For this review, take the finished solid that the model builds, in its own axes (mm). A direction names the side the tool comes from. Round coordinates to 2 decimals unless told otherwise and drop trailing zeros. Loops run counter-clockwise (first coordinate to the right, second up) from the corner with the lowest first, then second, coordinate; pieces in that order, holes last.
1) Mouldability with a two-part tool opening along Y and no side actions: class faces 1 (the flat face through (-5, 11, 0)), 2 (the flat face through (5, 20, 4)) as pulls with the +Y half, pulls with the -Y half, needs draft (parallel to the pull), parting line crosses it, or undercut.
2) Take a section at C-C (y = 19). State the section outline as (x, z) points.
3) Take a section at A-A (y = -20). State the section outline as (x, z) points, then the cut area to 3 significant figures.
4) Tool access review of faces 3 (the flat face through (-5, 11, 8)), 4 (the flat face through (-5, 20, 4)): name each direction out of +Z, -Z, +X, -X, +Y, -Y from which nothing blocks a thin tool from reaching the whole face with its end or side.
5) Wall thickness on L1, parallel to X at y = -20, z = 3.5; L2, parallel to Y at x = 0, z = 4.75 (3 decimals); L3, parallel to X at y = -6.5, z = 4.75: over which ranges is each line inside the solid? List them lowest first.
6) Insertion check: pin 1 (1.5 mm diameter, centred on y = 3, z = 2.5, fed in from +X); pin 2 (1 mm diameter, centred on x = 3.5, z = 2, fed in from -Y); pin 3 (4 mm diameter, centred on y = 22.5, z = 2, fed in from +X). Each pin has a flat end and moves straight along its axis. Give the tip position at first contact, or say it passes through.
7) Take a section at B-B (z = 5.25). Give the number of separate pieces and of enclosed holes in the cut face, then the cut area to 3 significant figures.
```python
from build123d import *

# Parameters (mm, degrees)
F1_DEPTH = 8
F3_COUNT = 3
F4_SIZE  = 0.762


with BuildPart() as f1:
    # F0 (on Top) → F1 (new body)
    with BuildSketch(Plane.XY):
        with BuildLine():
            ThreePointArc((-4.9999998882, 25.8578643368), (-2.5365296225, 25.2160215952), (0, 25))
            ThreePointArc((0, 25), (2.5365296809, 25.2160216052), (5, 25.8578643763))
            ThreePointArc((5, 25.8578643763), (12.2474487139, 31.3397459622), (15, 40))
            ThreePointArc((15, 40), (-8.6602540862, 52.2474486797), (-4.9999998882, 25.8578643368))
        make_face()
        with BuildLine():
            ThreePointArc((11.025, 40), (7.7958522626, 32.2041477374), (0, 28.975))
            ThreePointArc((0, 28.975), (-7.7958522626, 47.7958522626), (11.025, 40))
        make_face(mode=Mode.SUBTRACT)
        with BuildLine():
            Line((0, 25), (0, 15))
            ThreePointArc((0, 15), (2.5365296809, 14.7839783948), (5, 14.1421356237))
            Line((5, 14.1421356237), (5, 25.8578643763))
            ThreePointArc((5, 25.8578643763), (2.5365296809, 25.2160216052), (0, 25))
        make_face()
        with BuildLine():
            ThreePointArc((-4.9999998882, 14.1421356632), (-2.5365296225, 14.7839784048), (0, 15))
            Line((0, 15), (0, 25))
            ThreePointArc((0, 25), (-2.5365296225, 25.2160215952), (-4.9999998882, 25.8578643368))
            Line((-4.9999998882, 25.8578643368), (-4.9999998882, 14.1421356632))
        make_face()
        with BuildLine():
            ThreePointArc((5, 14.1421356237), (2.5365296809, 14.7839783948), (0, 15))
            ThreePointArc((0, 15), (-2.5365296225, 14.7839784048), (-4.9999998882, 14.1421356632))
            ThreePointArc((-4.9999998882, 14.1421356632), (-8.6602540862, -12.2474486797), (15, 0))
            ThreePointArc((15, 0), (12.2474487139, 8.6602540378), (5, 14.1421356237))
        make_face()
        with BuildLine():
            ThreePointArc((0, 11.025), (7.7958522626, 7.7958522626), (11.025, 0))
            ThreePointArc((11.025, 0), (-7.7958522626, -7.7958522626), (0, 11.025))
        make_face(mode=Mode.SUBTRACT)
    extrude(amount=F1_DEPTH)

    # F3: F1 ×3 about axis
    f3_axis = Axis((0, 0, 23.3244411647), (0, 0, 1))


with BuildPart() as f1_1:
    add(f1.part)
    for i in range(1, F3_COUNT):
        add(f1.part.rotate(f3_axis, i * 360 / F3_COUNT))

    # F4
    f4_edges = [f1_1.edges().sort_by_distance(p)[0] for p in [
        (0, 51.025, 8),
        (0, -11.025, 8),
        (-44.188946, -25.5125, 8),
        (44.188946, -25.5125, 8),
        (-44.188946, -25.5125, 0),
        (0, -11.025, 0),
        (44.188946, -25.5125, 0),
        (0, 51.025, 0),
    ]]
    chamfer(f4_edges, length=F4_SIZE)


solid = f1_1.part
```
Response:
1. face 1: needs draft
1. face 2: undercut
2. outline: (-5, 0) - (5, 0) - (5, 8) - (-5, 8) - close
3. outline: (-49.64, 0) - (-46.43, 0) - (-45.67, 0.76) - (-45.67, 7.24) - (-46.43, 8) - (-49.64, 8) - close; (-23.62, 0.76) - (-22.85, 0) - (-19.64, 0) - (-19.64, 8) - (-22.85, 8) - (-23.62, 7.24) - close; (19.64, 0) - (22.85, 0) - (23.62, 0.76) - (23.62, 7.24) - (22.85, 8) - (19.64, 8) - close; (45.67, 0.76) - (46.43, 0) - (49.64, 0) - (49.64, 8) - (46.43, 8) - (45.67, 7.24) - close
3. area: 125 mm2
4. face 3: +Z, +X, -X, +Y, -Y
4. face 4: +Z, -Z, -X
5. L1: x = -49.64 to -45.67, -23.62 to -19.64, 19.64 to 23.62, 45.67 to 49.64
5. L2: y = -15 to -11.025, 11.025 to 28.975, 51.025 to 55
5. L3: x = -41.18 to -28.1, -21.26 to -8.91, 8.91 to 21.26, 28.1 to 41.18
6. pin 1: stops at x = 14.83
6. pin 2: stops at y = -14.7
6. pin 3: stops at x = 5
7. separate pieces: 1
7. enclosed holes: 4
7. area: 1,620 mm2
